Read the model definition and answer for the solid it produces. Units are mm, in the model's axes. Round coordinates to 2 decimals unless told otherwise and drop trailing zeros. Loops run counter-clockwise (first coordinate to the right, second up) from the corner with the lowest first, then second, coordinate; pieces in that order, holes last. Notation, with made-up numbers: (-8.5, -33.5) - (9.5, -33.5) arc R24 ccw to (9.5, -20.5) - close; hole circle Ø6 at (78, -29.75). An arc over 180 degrees is marked (long way). Use one line per item in the form item = value. Start each with the question number.
```python
from build123d import *

# Parameters (mm, degrees)
SKETCH_1_R          = 4
EXTRUDE_1_DEPTH     = 2.2
SKETCH_2_R          = 1.5
CUT_EXTRUDE_1_DEPTH = 7
SKETCH_3_R          = 4.5
EXTRUDE_2_DEPTH     = 0.8
SKETCH_4_R          = 1.5
CUT_EXTRUDE_2_DEPTH = 0.8


with BuildPart() as part:
    # 草图1 → 凸台-拉伸1 (new body)
    with BuildSketch(Plane.XY):
        Circle(SKETCH_1_R)
    extrude(amount=EXTRUDE_1_DEPTH)

    # 草图2 → 切除-拉伸1 (cut)
    with BuildSketch(Plane.XY.offset(2.2)):
        Circle(SKETCH_2_R)
    extrude(amount=-CUT_EXTRUDE_1_DEPTH, mode=Mode.SUBTRACT)

    # 草图3 → 凸台-拉伸2 (add)
    with BuildSketch(Plane(origin=(0, 0, 0), x_dir=(-1, 0, 0), z_dir=(0, 0, -1))):
        Circle(SKETCH_3_R)
    extrude(amount=EXTRUDE_2_DEPTH)

    # 草图4 → 切除-拉伸2 (cut)
    with BuildSketch(Plane.XY):
        Circle(SKETCH_4_R)
    extrude(amount=-CUT_EXTRUDE_2_DEPTH, mode=Mode.SUBTRACT)


solid = part.part
```
1) Determine the mould class of faces 1 (the cylindrical face through (-1.5, 0.07, 0.72)), 2 (the cylindrical face through (-0.867, -3.905, 1.085)), 3 (the flat face through (3, -3, 0)) for opening direction X: +X half, -X half, draft (parallel to the pull), parting line (faces both ways), or undercut.
2) A cutting plane is placed at D-D on x = -2.75. Write down the section's boundary in (y, z).
3) Flat-ended cylindrical pins translate along their axes: pin 1 (1 mm diameter, centred on x = 1.5, z = 1.5, fed in from +Y); pin 2 (1.5 mm diameter, centred on x = -2.5, z = 1.5, fed in from -Y); pin 3 (1.5 mm diameter, centred on x = -3.5, z = 1, fed in from +Y). Find the tip coordinate at first contact, or state that the pin passes through.
4) Straight lines are drawn through the part: line 1 (Y direction, x = 0, z = 1.15); line 2 (X direction, y = -1.25, z = 0.95); line 3 (X direction, y = 0.75, z = 1.85). For each, find the intervals that lie inside material, in ascending order. Write a range as from..to.
5) A cutting plane is placed at C-C on z = 1.25. Write down the section's boundary in (x, y), plus the area to 3 significant figures.
6) A cutting plane is placed at A-A on y = 0. Write down the section's boundary in (x, z).
Checks:
q1.face_1 = undercut
q1.face_2 = parting line
q1.face_3 = draft
q2.outline = (-3.56, -0.8) - (3.56, -0.8) - (3.56, 0) - (2.9, 0) - (2.9, 2.2) - (-2.9, 2.2) - (-2.9, 0) - (-3.56, 0) - close
q3.pin_1 = 3.87
q3.pin_2 = -3.6
q3.pin_3 = 2.9
q4.line_1 = -4..-1.5, 1.5..4
q4.line_2 = -3.8..-0.83, 0.83..3.8
q4.line_3 = -3.93..-1.3, 1.3..3.93
q5.outline = circle Ø8 at (0, 0); hole circle Ø3 at (0, 0)
q5.area = 43.2 mm²
q6.outline = (-4.5, -0.8) - (-1.5, -0.8) - (-1.5, 2.2) - (-4, 2.2) - (-4, 0) - (-4.5, 0) - close; (1.5, -0.8) - (4.5, -0.8) - (4.5, 0) - (4, 0) - (4, 2.2) - (1.5, 2.2) - close
